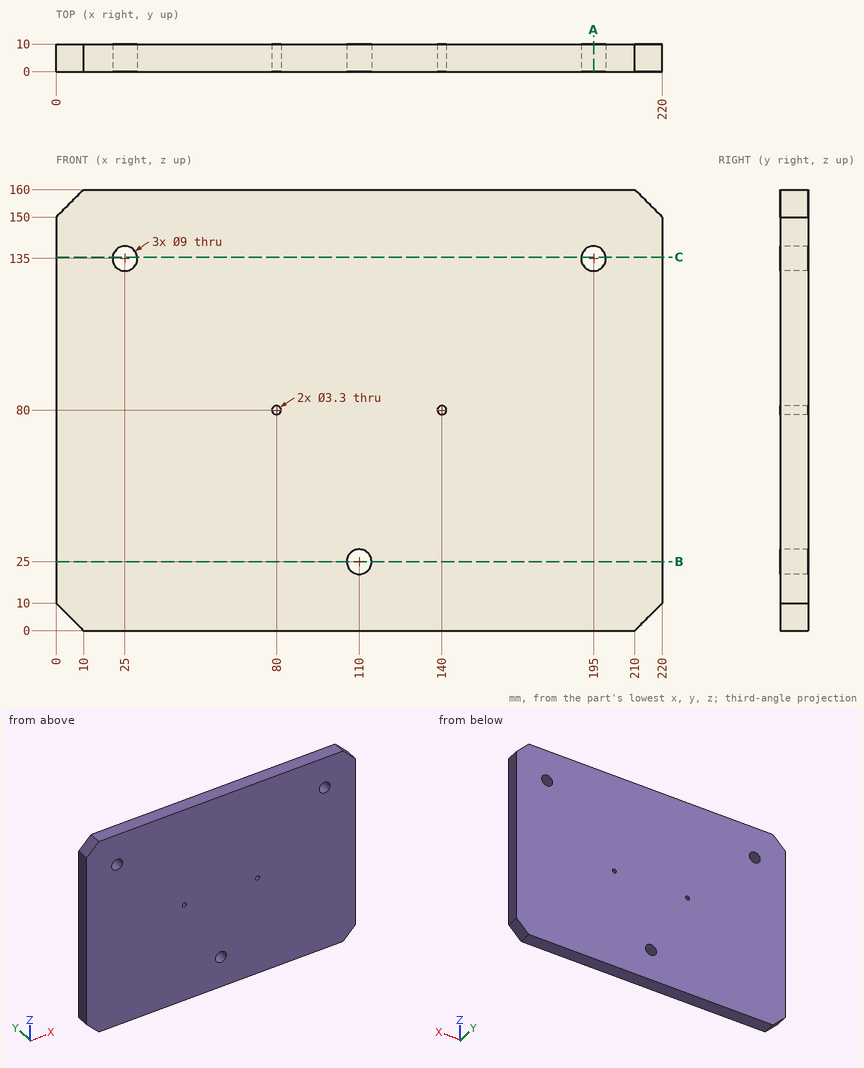
For this review, use the dimensioned drawing (mm, ordinates from the lowest corner) and the shaded views. Round coordinates to 2 decimals unless told otherwise and drop trailing zeros. Loops run counter-clockwise (first coordinate to the right, second up) from the corner with the lowest first, then second, coordinate; pieces in that order, holes last. Notation, with made-up numbers: M -24.75,-5.5 L 14.25,-5.5 A24 cw 14.25,10.5 Z; hole C 25,-39 d7. An arc over 180 degrees is marked long. Answer as a JSON object with one key per item and string values.
(1) Take a section at A-A on x = 195. Give the boundary of the cut face in (y, z).
Resolved:
{"outline": "M 0,0 L 10,0 L 10,130.5 L 0,130.5 Z; M 0,139.5 L 10,139.5 L 10,160 L 0,160 Z"}
(2) To check wall thickness, follow line 1 along X through (y, z) = (2.75, 135); line 2 along X through (y, z) = (3, 80); line 3 along Z through (x, y) = (80, 5.5). State the ranges of each line that lie inside material, in increasing order.
Resolved:
{"line 1": "0 to 20.5, 29.5 to 190.5, 199.5 to 220", "line 2": "0 to 78.35, 81.65 to 138.35, 141.65 to 220", "line 3": "0 to 78.35, 81.65 to 160"}
(3) Take a section at C-C on z = 135.5. Give the boundary of the cut face in (x, y).
Resolved:
{"outline": "M 0,0 L 20.53,0 L 20.53,10 L 0,10 Z; M 29.47,0 L 190.53,0 L 190.53,10 L 29.47,10 Z; M 199.47,0 L 220,0 L 220,10 L 199.47,10 Z"}
(4) Take a section at B-B on z = 25. Give the boundary of the cut face in (x, y).
Resolved:
{"outline": "M 0,0 L 105.5,0 L 105.5,10 L 0,10 Z; M 114.5,0 L 220,0 L 220,10 L 114.5,10 Z"}
